Check sheet for the modelled part. Datum: model origin and axes. Units: mm. A direction names the side the tool comes from. Give positions to 0.01 mm unless a question says otherwise; leave off trailing zeros. Loops run counter-clockwise (first coordinate to the right, second up) from the corner with the lowest first, then second, coordinate; pieces in that order, holes last. Notation, with made-up numbers: M 45,-23.75 L 87,-23.75 A27 cw 87,0.25 Z; hole C 81,85.5 d9. An arc over 180 degrees is marked long. Put each result on its own line as item: value. Start each with the question number.
```python
from build123d import *

# Parameters (mm, degrees)
SKETCH2_R           = 7
BOSS_EXTRUDE1_DEPTH = 8
BOSS_EXTRUDE2_DEPTH = 8
CIRPATTERN1_COUNT   = 17
SKETCH5_R           = 14.5
BOSS_EXTRUDE3_DEPTH = 13
SKETCH6_R           = 13.5
CUT_EXTRUDE1_DEPTH  = 11
SKETCH7_R           = 4
CUT_EXTRUDE2_DEPTH  = 11


with BuildPart() as part:
    # Sketch2 → Boss-Extrude1 (new body)
    with BuildSketch(Plane.XY):
        Circle(SKETCH2_R)
    extrude(amount=BOSS_EXTRUDE1_DEPTH)

    # Sketch4 → Boss-Extrude2 (add)
    with BuildSketch(Plane.XY):
        with BuildLine():
            Line((-0.95177028, 6.934993391), (-0.95177028, 7.934993391))
            Line((-0.95177028, 7.934993391), (-0.60177028, 9))
            Line((-0.60177028, 9), (0.39822972, 9))
            Line((0.39822972, 9), (0.74822972, 7.959895997))
            Line((0.74822972, 7.959895997), (0.74822972, 6.959895997))
            ThreePointArc((0.74822972, 6.959895997), (-0.102529141, 6.999249087), (-0.95177028, 6.934993391))
        make_face()
    boss_extrude2 = extrude(amount=BOSS_EXTRUDE2_DEPTH)

    # CirPattern1: Boss-Extrude2 ×17 about axis
    cirpattern1_axis = Axis((0, 0, 0), (0, 0, 1))
    for i in range(1, CIRPATTERN1_COUNT):
        add(boss_extrude2.rotate(cirpattern1_axis, i * 360 / CIRPATTERN1_COUNT))

    # Sketch5 → Boss-Extrude3 (add)
    with BuildSketch(Plane(origin=(0, 0, 0), x_dir=(-1, 0, 0), z_dir=(0, 0, -1))):
        with Locations(Location((0, 0, 0), (0, 0, 180))):
            Circle(SKETCH5_R)
    extrude(amount=BOSS_EXTRUDE3_DEPTH)

    # Sketch6 → Cut-Extrude1 (cut)
    with BuildSketch(Plane(origin=(0, 0, -13), x_dir=(-1, 0, 0), z_dir=(0, 0, -1))):
        Circle(SKETCH6_R)
    extrude(amount=-CUT_EXTRUDE1_DEPTH, mode=Mode.SUBTRACT)

    # Sketch7 → Cut-Extrude2 (cut)
    with BuildSketch(Plane.XY.offset(8)):
        Circle(SKETCH7_R)
    extrude(amount=-CUT_EXTRUDE2_DEPTH, mode=Mode.SUBTRACT)


solid = part.part
```
Q1. Mould release check, pull along Y, two halves, no side actions. Record for faces 1 (the face through (-2.44, -6.56, 3.94)), 2 (the face through (8.504, 0.215, 3.944)), 3 (the face through (3.983, -7.516, 3.944)), 4 (the face through (-5.3, 6.66, 3.94)): pulls with the +Y half, pulls with the -Y half, needs draft (parallel to the pull), parting line crosses it, or undercut.
Q2. Thickness scan on line 1 along Y through (x, z) = (0, -8); line 2 along Y through (x, z) = (0, 2); line 3 along Z through (x, y) = (13, -2.25). Record the ranges inside material, lowest first. Write a range as [from, to].
Q3. Section check A-A, the plane y = 10.25. Record the cut outline in (x, z).
Q4. Depth check by flat-ended pin: P1, Ø4, axis at y = 4, z = -10, coming from the -X side; P2, Ø0.5, axis at x = 0, z = 5, coming from the +Y side; P3, Ø6, axis at y = 4, z = 2, coming from the +X side. Enter the tip coordinate at first touch or a pass-through.
Q5. Section check C-C, the plane x = -9.75. Record the cut outline in (y, z), then the cut area to 3 significant figures.
Q6. Section check B-B, the plane z = -6. Record the cut outline in (x, y).
Q7. Access from +Z, -Z, +X, -X, +Y, -Y to the whole of each face (thin tool, end or side, straight path). Record for faces 5 (the face through (3, -7, 0)), 6 (the face through (6.43, -5.57, 3.94)), 7 (the face through (-7.387, -1.324, 3.944)).
Found:
1. face 1: undercut
1. face 2: undercut
1. face 3: pulls with the -Y half
1. face 4: pulls with the +Y half
2. line 1: y = [-14.5, -13.5], [13.5, 14.5]
2. line 2: y = [-7, -4], [4, 9]
2. line 3: z = [-2, 0]
3. outline: M -10.26,-13 L -8.79,-13 L -8.79,-2 L 8.79,-2 L 8.79,-13 L 10.26,-13 L 10.26,0 L -10.26,0 Z
4. P1: stops at x = -14.36
4. P2: stops at y = 9
4. P3: stops at x = 14.39
5. outline: M -10.73,-13 L -9.34,-13 L -9.34,-2 L 9.34,-2 L 9.34,-13 L 10.73,-13 L 10.73,0 L -10.73,0 Z
5. area: 73.6 mm^2
6. outline: C 0,0 d29; hole C 0,0 d27
7. face 5: +Z
7. face 6: +Z, -Y
7. face 7: +Z, -X
